```python
from build123d import *

# Parameters (mm, degrees)
SKETCH_1_R      = 0.8
EXTRUDE_2_DEPTH = 1
SKETCH_2_R      = 0.8
SKETCH_2_W      = 4
SKETCH_2_H      = 2
SKETCH_2_W_2    = 2.4
SKETCH_2_H_2    = 1.5
EXTRUDE_3_DEPTH = 0.01


with BuildPart() as part:
    # 草图1 → 凸台-拉伸2 (new body)
    with BuildSketch(Plane.XY):
        Polygon((0, 13.3), (0, 0), (14, 0), (14, 13.3), (8, 13.3), (8, 11.3), (6, 11.3), (6, 13.3), align=None)
        with Locations((1.4, 1.4)):
            Circle(SKETCH_1_R, mode=Mode.SUBTRACT)
        with Locations((12.6, 1.4)):
            Circle(SKETCH_1_R, mode=Mode.SUBTRACT)
        with Locations((1.4, 11.9)):
            Circle(SKETCH_1_R, mode=Mode.SUBTRACT)
        with Locations((12.6, 11.9)):
            Circle(SKETCH_1_R, mode=Mode.SUBTRACT)
    extrude(amount=EXTRUDE_2_DEPTH)

    # 草图2 → 凸台-拉伸3 (add)
    with BuildSketch(Plane.XY.offset(1)):
        Polygon((0, 0), (14, 0), (14, 13.3), (8, 13.3), (8, 11.3), (6, 11.3), (6, 13.3), (0, 13.3), align=None)
        with Locations((1.4, 1.4)):
            Circle(SKETCH_2_R, mode=Mode.SUBTRACT)
        with Locations((2.2, 4.65)):
            Rectangle(SKETCH_2_W, SKETCH_2_H, mode=Mode.SUBTRACT)
        with Locations((7, 1.6)):
            Rectangle(SKETCH_2_W_2, SKETCH_2_H, mode=Mode.SUBTRACT)
        with Locations((12.6, 1.4)):
            Circle(SKETCH_2_R, mode=Mode.SUBTRACT)
        with Locations((11.8, 3.65)):
            Rectangle(SKETCH_2_W, SKETCH_2_H_2, mode=Mode.SUBTRACT)
        with Locations((11.8, 5.65)):
            Rectangle(SKETCH_2_W, SKETCH_2_H_2, mode=Mode.SUBTRACT)
        with Locations((2.2, 8.65)):
            Rectangle(SKETCH_2_W, SKETCH_2_H, mode=Mode.SUBTRACT)
        with Locations((1.4, 11.9)):
            Circle(SKETCH_2_R, mode=Mode.SUBTRACT)
        with Locations((11.8, 7.65)):
            Rectangle(SKETCH_2_W, SKETCH_2_H_2, mode=Mode.SUBTRACT)
        with Locations((11.8, 9.65)):
            Rectangle(SKETCH_2_W, SKETCH_2_H_2, mode=Mode.SUBTRACT)
        with Locations((7, 10)):
            Rectangle(SKETCH_2_W_2, SKETCH_2_H, mode=Mode.SUBTRACT)
        with Locations((12.6, 11.9)):
            Circle(SKETCH_2_R, mode=Mode.SUBTRACT)
    extrude(amount=EXTRUDE_3_DEPTH)


solid = part.part
```
Here's how the part is built. I have some questions about the finished solid (model axes, mm). A direction names the side the tool comes from. Give positions to 0.01 mm unless a question says otherwise; leave off trailing zeros. Loops run counter-clockwise (first coordinate to the right, second up) from the corner with the lowest first, then second, coordinate; pieces in that order, holes last. Notation, with made-up numbers: (69, 44.5) -> (117, 44.5) arc R11 ccw to (117, 63.5) -> close; hole circle Ø2 at (-30, -32). An arc over 180 degrees is marked (long way). Use one line per item in the form item = value. Start each with the question number.
1) Which directions (+Z, -Z, +X, -X, +Y, -Y) give clear straight access to the entire face, cutting with the end or side of a thin tool? Please do faces 5 (the face through (7, 7, 0)), 6 (the face through (7, 11.3, 0.5)).
2) Imagine slicing it at C-C (z = 0.45). Please give me the cut outline in (x, y), then the cut area to 3 significant figures.
3) Imagine slicing it at A-A (y = 1.4). Count the separate pieces of the cut face and the enclosed holes in it, then the cut area to 3 significant figures.
4) Please list where these lines run through material, in increasing order: line 1 along Y through (x, z) = (1.4, 0.65); line 2 along X through (y, z) = (2, 0.75); line 3 along Z through (x, y) = (13, 7.25).
5) Thinking about a two-plate mould opening in Y: for faces 1 (the face through (1.296, 12.693, 0.498)), 2 (the face through (3, 13.3, 0.5)), 3 (the face through (1.83, 2.075, 0.498)), 4 (the face through (6.9, 0, 0.5)), which applies, +Y half, -Y half, draft (parallel to the pull), parting line (faces both ways), or undercut?
Check values:
q1.face_5 = -Z, +X, -X, +Y, -Y
q1.face_6 = +Z, -Z, +Y
q2.outline = (0, 0) -> (14, 0) -> (14, 13.3) -> (8, 13.3) -> (8, 11.3) -> (6, 11.3) -> (6, 13.3) -> (0, 13.3) -> close; hole circle Ø1.6 at (1.4, 1.4); hole circle Ø1.6 at (1.4, 11.9); hole circle Ø1.6 at (12.6, 1.4); hole circle Ø1.6 at (12.6, 11.9)
q2.area = 174 mm^2
q3.separate_pieces = 3
q3.enclosed_holes = 0
q3.area = 10.9 mm^2
q4.line_1 = 0 to 0.6, 2.2 to 11.1, 12.7 to 13.3
q4.line_2 = 0 to 0.87, 1.93 to 12.07, 13.13 to 14
q4.line_3 = 0 to 1
q5.face_1 = undercut
q5.face_2 = +Y half
q5.face_3 = undercut
q5.face_4 = -Y half
